Study the drawing (mm; zero at the part's minimum x, y, z) and answer. Round coordinates to 2 decimals unless told otherwise and drop trailing zeros. Write each loop counter-clockwise with the first axis right and the second up, starting at its lowest first coordinate (ties: lowest second). Pieces come first, ordered by that corner, then holes. Notation, with made-up numbers: (11, -1) - (30, -1) arc R28 cw to (30, 32) - close; hole circle Ø9 at (25.5, -29.75). An arc over 180 degrees is marked (long way). Use one line per item in the form item = value. Start each with the question number.
1) The part is cut by section A-A, the plane z = 40. Give the vertices of the cut face in (x, y), plus the area to 3 significant figures.
2) The part is cut by section B-B, the plane y = 1.95. Give the vertices of the cut face in (x, z) (1 decimal).
3) The part is cut by section D-D, the plane z = 29. Give the vertices of the cut face in (x, y).
4) Each of these flat-tipped pins is pushed along its axis until it touches: pin 1 (1.5 mm diameter, centred on y = 1, z = 13, fed in from +X); pin 2 (0.9 mm diameter, centred on x = 85.5, y = 2, fed in from -Z); pin 3 (0.9 mm diameter, centred on x = 76.5, y = 1.5, fed in from +Z). Where does it stop, or does it pass through?
5) Consider line 1 along X through (y, z) = (0.7, 32); line 2 along X through (y, z) = (0.6, 18); line 3 along Z through (x, y) = (27, 0.55). Determine where each line is inside the solid, lowest interval first. Write a range as from..to.
6) The part is cut by section C-C, the plane x = 13. Give the vertices of the cut face in (y, z).
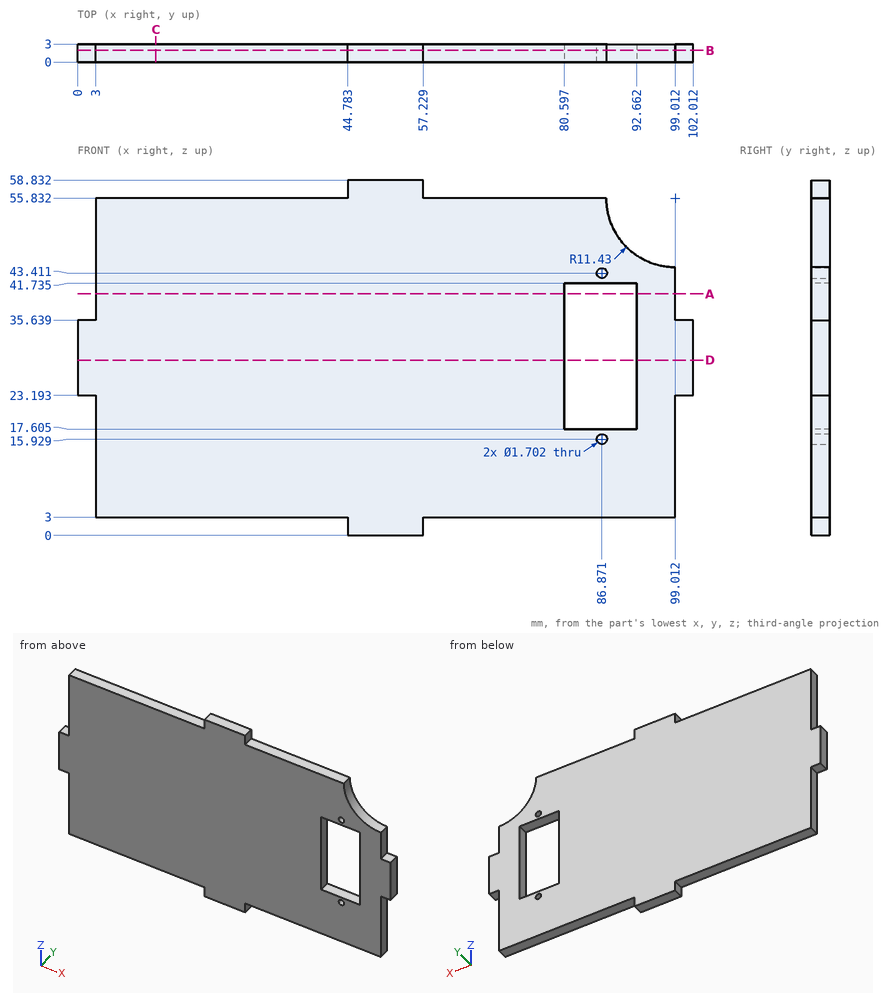
Geometry results:
q1.outline = (3, 0) - (80.6, 0) - (80.6, 3) - (3, 3) - close; (92.66, 0) - (99.01, 0) - (99.01, 3) - (92.66, 3) - close
q1.area = 252 mm2
q2.outline = (0, 23.2) - (3, 23.2) - (3, 3) - (44.8, 3) - (44.8, 0) - (57.2, 0) - (57.2, 3) - (99, 3) - (99, 23.2) - (102, 23.2) - (102, 35.6) - (99, 35.6) - (99, 44.4) arc R11.4 cw to (87.6, 55.8) - (57.2, 55.8) - (57.2, 58.8) - (44.8, 58.8) - (44.8, 55.8) - (3, 55.8) - (3, 35.6) - (0, 35.6) - close; hole (80.6, 17.6) - (92.7, 17.6) - (92.7, 41.7) - (80.6, 41.7) - close; hole circle Ø1.7 at (86.9, 15.9); hole circle Ø1.7 at (86.9, 43.4)
q3.outline = (0, 0) - (80.6, 0) - (80.6, 3) - (0, 3) - close; (92.66, 0) - (102.01, 0) - (102.01, 3) - (92.66, 3) - close
q4.pin_1 = 99.01
q4.pin_2 = 3
q4.pin_3 = 55.83
q5.line_1 = 0..80.6, 92.66..102.01
q5.line_2 = 3..80.6, 92.66..99.01
q5.line_3 = 3..55.83
q6.outline = (0, 3) - (3, 3) - (3, 55.83) - (0, 55.83) - close
